Could you check a few things on this model? Use its own coordinates, in mm. A direction names the side the tool comes from. Give positions to 0.01 mm unless a question says otherwise; leave off trailing zeros. Loops run counter-clockwise (first coordinate to the right, second up) from the corner with the lowest first, then second, coordinate; pieces in that order, holes last. Notation, with made-up numbers: M -28.75,4 L -24.75,4 A28 cw -24.75,29 Z; hole C -19,81.25 d10. An arc over 180 degrees is marked long. Use a Markdown table: item, result. Add a question column.
1) If I drill on line 1 along Z through (x, y) = (9, -8); line 2 along Z through (x, y) = (11, -17); line 3 along Y through (x, z) = (7.5, 20), over which ranges is the centre line in solid material (lowest first)? Write a range as [from, to].
2) Which directions (+Z, -Z, +X, -X, +Y, -Y) give clear straight access to the entire face, cutting with the end or side of a thin tool? Please do faces 1 (the flat face through (-10.25, -5, 20)), 2 (the flat face through (10.25, -5, 20)), 3 (the flat face through (2, -4, 19)), 4 (the flat face through (-1, -19.75, 0)).
3) Will these pins go through, and if not, where does the flat tip stop? pin 1 Ø1.5 at (y, z) = (-2.5, -20.5) entering from +X; pin 2 Ø6 at (y, z) = (-41, -15.5) entering from +X; pin 3 Ø4 at (y, z) = (-10, -16) entering from +X.
4) Suppose I cut it at B-B on x = 12.5. List the corners of the cut face in (y, z) for me.
5) Suppose I cut it at D-D on y = -35. List the corners of the cut face in (x, z) for me, and give its area (3 significant figures).
6) Suppose I cut it at A-A on z = 14. List the corners of the cut face in (x, y) for me, and give its area (3 significant figures).
7) Suppose I cut it at C-C on x = 0. Count the separate pieces of the cut face and the enclosed holes in it, and give its area (3 significant figures).
8) We'd pull the mould along Z, two halves only. Please class faces 5 (the flat face through (2, -4, -19)), 6 (the flat face through (10.25, -5, -21)), 7 (the flat face through (-1, -30, -22)): +Z half, -Z half, draft (parallel to the pull), parting line (faces both ways), or undercut.
```python
from build123d import *

# Parameters (mm, degrees)
BOSS_EXTRUDE1_DEPTH      = 22
BOSS_EXTRUDE1_DEPTH_BACK = 22
SKETCH2_W                = 38
SKETCH2_H                = 20
CUT_EXTRUDE1_DEPTH       = 105.423416914
SKETCH3_W                = 7
SKETCH3_H                = 44
BOSS_EXTRUDE2_DEPTH      = 65.5
SKETCH23_R               = 5
SKETCH23_R_2             = 1.2
CUT_EXTRUDE2_DEPTH       = 111.605436123
SKETCH24_W               = 28.5
SKETCH24_H               = 34
CUT_EXTRUDE3_DEPTH       = 90.954502389
SKETCH26_R               = 1.2
SKETCH26_R_2             = 5
SKETCH26_R_3             = 1.45
CUT_EXTRUDE6_DEPTH       = 107.330263801
SKETCH27_W               = 29.7
SKETCH27_H               = 35.2
CUT_EXTRUDE8_DEPTH       = 73.137455597
SKETCH29_W               = 7
SKETCH29_H               = 30
CUT_EXTRUDE10_DEPTH      = 74.468530678
CHAMFER2_SIZE            = 5
BOSS_EXTRUDE4_DEPTH      = 22
BOSS_EXTRUDE4_DEPTH_BACK = 22
SKETCH31_W               = 28.5
SKETCH31_H               = 34
CUT_EXTRUDE11_DEPTH      = 10
FILLET1_R                = 10


with BuildPart() as part:
    # Sketch1 → Boss-Extrude1 (new, two sides: drawn at the far end of the back side and taken through both)
    with BuildSketch(Plane.XY.offset(-BOSS_EXTRUDE1_DEPTH_BACK)):
        with BuildLine():
            Line((10.25, -60), (10.25, 0))
            ThreePointArc((10.25, 0), (0, -10.25), (-10.25, 0))
            Line((-10.25, 0), (-10.25, -60))
            Line((-10.25, -60), (-10.25, -100))
            Line((-10.25, -100), (10.25, -100))
            Line((10.25, -100), (10.25, -60))
        make_face()
        with BuildLine():
            Line((10.25, 0), (9.2, 0))
            ThreePointArc((9.2, 0), (8.816088231, -0.879772698), (7.91, -1.196620241))
            ThreePointArc((7.91, -1.196620241), (5.656854249, -5.656854249), (1.196620241, -7.91))
            ThreePointArc((1.196620241, -7.91), (1.199154762, -7.954968281), (1.2, -8))
            ThreePointArc((1.2, -8), (-0.045031719, -9.199154762), (-1.196620241, -7.91))
            ThreePointArc((-1.196620241, -7.91), (-5.656854249, -5.656854249), (-7.91, -1.196620241))
            ThreePointArc((-7.91, -1.196620241), (-8.816088231, -0.879772698), (-9.2, 0))
            Line((-9.2, 0), (-10.25, 0))
            ThreePointArc((-10.25, 0), (0, -10.25), (10.25, 0))
        make_face()
        with BuildLine():
            ThreePointArc((7.91, -1.196620241), (7.120227302, -0.816088231), (6.8, 0))
            Line((6.8, 0), (4.2, 0))
            ThreePointArc((4.2, 0), (0, -4.2), (-4.2, 0))
            Line((-4.2, 0), (-6.8, 0))
            ThreePointArc((-6.8, 0), (-7.120227302, -0.816088231), (-7.91, -1.196620241))
            ThreePointArc((-7.91, -1.196620241), (-5.656854249, -5.656854249), (-1.196620241, -7.91))
            ThreePointArc((-1.196620241, -7.91), (0, -6.8), (1.196620241, -7.91))
            ThreePointArc((1.196620241, -7.91), (5.656854249, -5.656854249), (7.91, -1.196620241))
        make_face()
        with BuildLine():
            Line((4.2, 0), (6.8, 0))
            ThreePointArc((6.8, 0), (7.120227302, 0.816088231), (7.91, 1.196620241))
            ThreePointArc((7.91, 1.196620241), (5.656854249, 5.656854249), (1.196620241, 7.91))
            ThreePointArc((1.196620241, 7.91), (0, 6.8), (-1.196620241, 7.91))
            ThreePointArc((-1.196620241, 7.91), (-5.656854249, 5.656854249), (-7.91, 1.196620241))
            ThreePointArc((-7.91, 1.196620241), (-7.120227302, 0.816088231), (-6.8, 0))
            Line((-6.8, 0), (-4.2, 0))
            ThreePointArc((-4.2, 0), (0, 4.2), (4.2, 0))
        make_face()
        with BuildLine():
            ThreePointArc((7.91, 1.196620241), (8.816088231, 0.879772698), (9.2, 0))
            Line((9.2, 0), (10.25, 0))
            ThreePointArc((10.25, 0), (0, 10.25), (-10.25, 0))
            Line((-10.25, 0), (-9.2, 0))
            ThreePointArc((-9.2, 0), (-8.816088231, 0.879772698), (-7.91, 1.196620241))
            ThreePointArc((-7.91, 1.196620241), (-5.656854249, 5.656854249), (-1.196620241, 7.91))
            ThreePointArc((-1.196620241, 7.91), (-0.045031719, 9.199154762), (1.2, 8))
            ThreePointArc((1.2, 8), (1.199154762, 7.954968281), (1.196620241, 7.91))
            ThreePointArc((1.196620241, 7.91), (5.656854249, 5.656854249), (7.91, 1.196620241))
        make_face()
    extrude(amount=BOSS_EXTRUDE1_DEPTH + BOSS_EXTRUDE1_DEPTH_BACK)

    # Sketch2 → Cut-Extrude1 (cut, through all)
    with BuildSketch(Plane.ZY.offset(10.25)):
        with Locations((0, 0.25)):
            Rectangle(SKETCH2_W, SKETCH2_H)
    extrude(amount=-CUT_EXTRUDE1_DEPTH, mode=Mode.SUBTRACT)

    # Sketch3 → Boss-Extrude2 (add)
    with BuildSketch(Plane(origin=(0, -9.75, 0), x_dir=(1, 0, 0), z_dir=(0, 1, 0))):
        with Locations((-13.75, 0)):
            Rectangle(SKETCH3_W, SKETCH3_H)
        with Locations((13.75, 0)):
            Rectangle(SKETCH3_W, SKETCH3_H)
    extrude(amount=-BOSS_EXTRUDE2_DEPTH)

    # Sketch23 → Cut-Extrude2 (cut, through all)
    with BuildSketch(Plane.XY.offset(22)):
        with BuildLine():
            Line((-10.25, -100), (10.25, -100))
            Line((10.25, -100), (10.25, -85))
            ThreePointArc((10.25, -85), (0, -95.25), (-10.25, -85))
            Line((-10.25, -85), (-10.25, -100))
        make_face()
        with Locations((0, -85)):
            Circle(SKETCH23_R)
        with Locations((8, -85)):
            Circle(SKETCH23_R_2)
        with Locations((0, -77)):
            Circle(SKETCH23_R_2)
        with Locations((0, -93)):
            Circle(SKETCH23_R_2)
        with Locations((-8, -85)):
            Circle(SKETCH23_R_2)
    extrude(amount=-CUT_EXTRUDE2_DEPTH, mode=Mode.SUBTRACT)

    # Sketch24 → Cut-Extrude3 (cut, through all)
    with BuildSketch(Plane(origin=(0, -9.75, 0), x_dir=(1, 0, 0), z_dir=(0, 1, 0))):
        Rectangle(SKETCH24_W, SKETCH24_H)
    extrude(amount=-CUT_EXTRUDE3_DEPTH, mode=Mode.SUBTRACT)

    # Sketch26 → Cut-Extrude6 (cut, through all)
    # profile 1 of 5: a face of its own
    with BuildSketch(Plane.XY.offset(22)):
        with BuildLine():
            Line((10.25, -75.25), (14.25, -75.25))
            Line((14.25, -75.25), (14.25, -56.53282359))
            Line((14.25, -56.53282359), (14.25, -56.25))
            Line((14.25, -56.25), (-14.25, -56.25))
            Line((-14.25, -56.25), (-14.25, -56.53282359))
            Line((-14.25, -56.53282359), (-14.25, -75.25))
            Line((-14.25, -75.25), (-10.25, -75.25))
            Line((-10.25, -75.25), (-10.25, -85))
            ThreePointArc((-10.25, -85), (0, -95.25), (10.25, -85))
            Line((10.25, -85), (10.25, -75.25))
        make_face()
        with Locations((-8, -85)):
            Circle(SKETCH26_R, mode=Mode.SUBTRACT)
        with Locations((0, -85)):
            Circle(SKETCH26_R_2, mode=Mode.SUBTRACT)
        with Locations((0, -77)):
            Circle(SKETCH26_R, mode=Mode.SUBTRACT)
        with Locations((0, -93)):
            Circle(SKETCH26_R, mode=Mode.SUBTRACT)
        with Locations((8, -85)):
            Circle(SKETCH26_R, mode=Mode.SUBTRACT)
    # profile 2 of 5: a face of its own
    with BuildSketch(Plane.XY.offset(22)):
        Polygon((-17.25, -75.25), (-14.25, -75.25), (-14.25, -56.53282359), (-14.25, -56.25), (-17.25, -56.25), align=None)
    # profile 3 of 5: a face of its own
    with BuildSketch(Plane.XY.offset(22)):
        Polygon((14.25, -56.53282359), (14.25, -75.25), (17.25, -75.25), (17.25, -56.25), (14.25, -56.25), align=None)
    # profile 4 of 5: a face of its own
    with BuildSketch(Plane.XY.offset(22)):
        with Locations((-11, -53)):
            Circle(SKETCH26_R_3)
    # profile 5 of 5: a face of its own
    with BuildSketch(Plane.XY.offset(22)):
        with Locations((11, -53)):
            Circle(SKETCH26_R_3)
    extrude(amount=-CUT_EXTRUDE6_DEPTH, mode=Mode.SUBTRACT)

    # Sketch27 → Cut-Extrude8 (cut, through all)
    with BuildSketch(Plane.XZ.offset(56.25)):
        Rectangle(SKETCH27_W, SKETCH27_H)
    extrude(amount=-CUT_EXTRUDE8_DEPTH, mode=Mode.SUBTRACT)

    # Sketch29 → Cut-Extrude10 (cut, through all)
    with BuildSketch(Plane(origin=(0, 0, -22), x_dir=(-1, 0, 0), z_dir=(0, 0, -1))):
        with Locations((-13.75, -24.75)):
            Rectangle(SKETCH29_W, SKETCH29_H)
    extrude(amount=-CUT_EXTRUDE10_DEPTH, mode=Mode.SUBTRACT)

    # Chamfer2
    # the kernel refuses this chamfer: 5 mm, written as the material it takes off along each edge
    with BuildSketch(Plane(origin=(-17.25, -56.25, 34.85841494), x_dir=(0.9996219169112968, -0.027495876610586327, 0), z_dir=(0, 0, -1))) as chamfer2_piece_1:
        Polygon((CHAMFER2_SIZE * 0.999621916911, -CHAMFER2_SIZE * 0.0274958766106), (-CHAMFER2_SIZE * 0.0274958766106, -CHAMFER2_SIZE * 0.999621916911), (0, 0), align=None)
    extrude(amount=69.71682988, mode=Mode.SUBTRACT)

    # Sketch30 → Boss-Extrude4 (add, two sides: drawn at the far end of the back side and taken through both)
    with BuildSketch(Plane.XY.offset(-BOSS_EXTRUDE4_DEPTH_BACK)):
        Polygon((24.75, -56.25), (17.25, -32.198275862), (17.25, -56.25), align=None)
        Polygon((17.25, -32.198275862), (10.25, -9.75), (-17.25, -9.75), (-17.25, -56.25), (17.25, -56.25), align=None)
    extrude(amount=BOSS_EXTRUDE4_DEPTH + BOSS_EXTRUDE4_DEPTH_BACK)

    # Sketch31 → Cut-Extrude11 (cut)
    with BuildSketch(Plane(origin=(0, -9.75, 0), x_dir=(1, 0, 0), z_dir=(0, 1, 0))):
        Rectangle(SKETCH31_W, SKETCH31_H)
    extrude(amount=-CUT_EXTRUDE11_DEPTH, mode=Mode.SUBTRACT)

    # Fillet1
    fillet1_edges = [part.edges().sort_by_distance(p)[0] for p in [
        (-17.25, -56.25, 0),
    ]]
    fillet(fillet1_edges, radius=FILLET1_R)


solid = part.part
```
Answer block:
| question | item | result |
|---|---|---|
| 1 | line 1 | z = [-22, -19], [19, 22] |
| 1 | line 2 | z = [-22, -17], [17, 22] |
| 1 | line 3 | y = [-56.25, -1.09], [1.09, 6.99] |
| 2 | face 1 | +Z, -Z, -X, +Y |
| 2 | face 2 | +Z, -Z, +X, +Y |
| 2 | face 3 | +X, -X, +Y |
| 2 | face 4 | +X, +Y |
| 3 | pin 1 | stops at x = 10.25 |
| 3 | pin 2 | stops at x = 20.93 |
| 3 | pin 3 | stops at x = 10.87 |
| 4 | outline | M -56.25,-22 L -16.97,-22 L -16.97,-17 L -19.75,-17 L -19.75,17 L -16.97,17 L -16.97,22 L -56.25,22 Z |
| 5 | outline | M -17.25,-22 L 18.12,-22 L 18.12,22 L -17.25,22 Z |
| 5 | area | 1,560 mm^2 |
| 6 | outline | M -17.25,-46.25 A10 ccw -7.25,-56.25 L 24.75,-56.25 L 13.37,-19.75 L -14.25,-19.75 L -14.25,-9.75 L -17.25,-9.75 Z |
| 6 | area | 1,330 mm^2 |
| 7 | separate pieces | 7 |
| 7 | enclosed holes | 0 |
| 7 | area | 1,750 mm^2 |
| 8 | face 5 | undercut |
| 8 | face 6 | draft |
| 8 | face 7 | -Z half |
